Design review of the part shown in the three views and the two pictorial views. Dimensions are in mm from the part's minimum x, y and z. A direction names the side the tool comes from. Coordinates: 2 decimals unless noted, no trailing zeros. Loops run counter-clockwise (first coordinate to the right, second up) from the corner with the lowest first, then second, coordinate; pieces in that order, holes last. Notation, with made-up numbers: (-9, 38) -> (4, 38) arc R31 cw to (4, 67) -> close; hole circle Ø7 at (19.5, 14.25). An arc over 180 degrees is marked (long way). One line per item, written item: value. Start each with the question number.
1. Add section B-B on z = 14. Write out the cut boundary in (x, y).
2. Insertion check: pin 1 (1.5 mm diameter, centred on x = 21, z = 7, fed in from -Y); pin 2 (6 mm diameter, centred on x = 5, y = 28, fed in from +Z). Each pin has a flat end and moves straight along its axis. Give the tip position at first contact, or say it passes through.
3. Add section C-C on y = 21. Write out the cut boundary in (x, z).
4. Add section D-D on z = 31. Write out the cut boundary in (x, y).
5. For probe 1 along Y at (x, z) = (5.25, 14); probe 2 along X at (y, z) = (0.5, 32); probe 3 along Z at (x, y) = (16.75, 49.5), list the stretches that pass through material, from the lowest coordinate up.
6. Machinability: for the marked faces 1 and 2, which of the approach directions +Z, -Z, +X, -X, +Y, -Y give a long, thin tool a straight path to every point of the face, cutting with its end or side? Answer none if there is none.
7. Draft analysis for pull direction Y (two halves, no side actions). For the marked faces 3, 4 and 5, state which applies: pulls with the +Y half, pulls with the -Y half, needs draft (parallel to the pull), parting line crosses it, or undercut.
8. Add section A-A on x = 5.5. Write out the cut boundary in (y, z), plus the area to 3 significant figures.
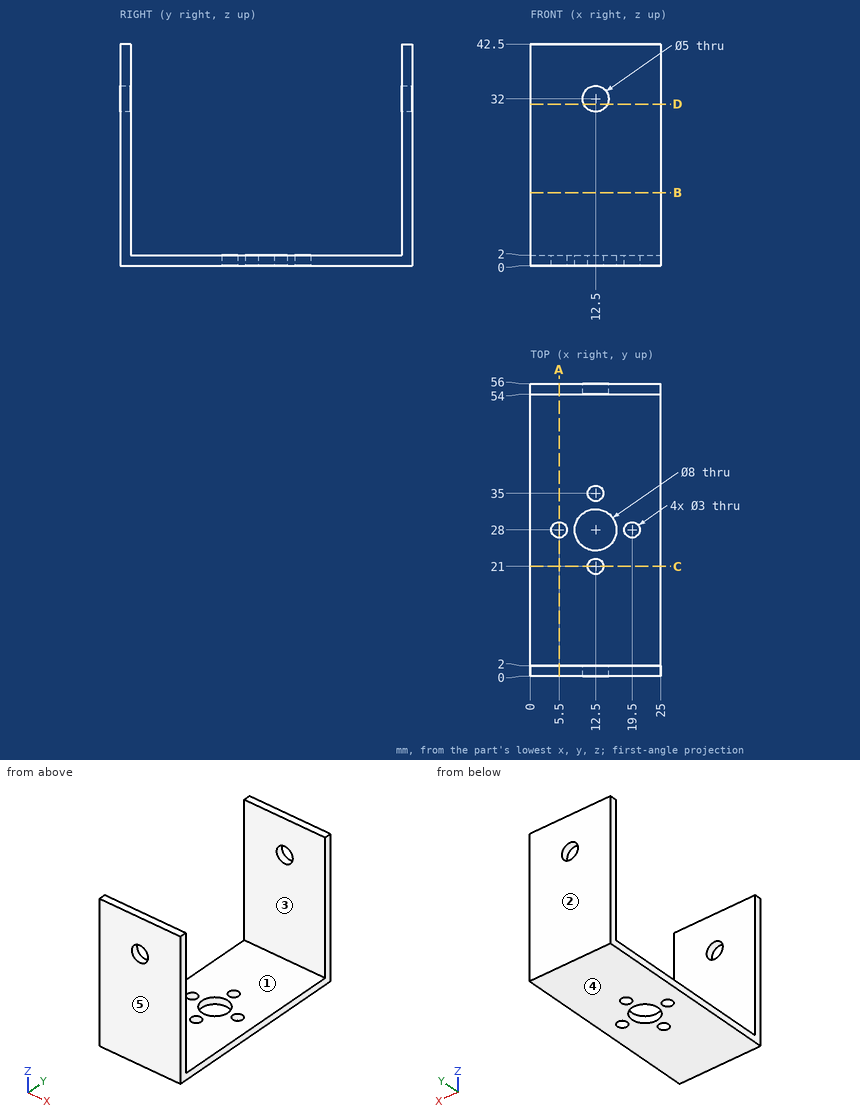
Worked answers:
1. outline: (0, 0) -> (25, 0) -> (25, 2) -> (0, 2) -> close; (0, 54) -> (25, 54) -> (25, 56) -> (0, 56) -> close
2. pin 1: stops at y = 0
2. pin 2: stops at z = 2
3. outline: (0, 0) -> (11, 0) -> (11, 2) -> (0, 2) -> close; (14, 0) -> (25, 0) -> (25, 2) -> (14, 2) -> close
4. outline: (0, 0) -> (10.21, 0) -> (10.21, 2) -> (0, 2) -> close; (0, 54) -> (10.21, 54) -> (10.21, 56) -> (0, 56) -> close; (14.79, 0) -> (25, 0) -> (25, 2) -> (14.79, 2) -> close; (14.79, 54) -> (25, 54) -> (25, 56) -> (14.79, 56) -> close
5. probe 1: y = 0 to 2, 54 to 56
5. probe 2: x = 0 to 10, 15 to 25
5. probe 3: z = 0 to 2
6. face 1: +Z, +X, -X
6. face 2: +Z, -Z, +X, -X, +Y
7. face 3: undercut
7. face 4: needs draft
7. face 5: pulls with the -Y half
8. outline: (0, 0) -> (26.5, 0) -> (26.5, 2) -> (2, 2) -> (2, 42.5) -> (0, 42.5) -> close; (29.5, 0) -> (56, 0) -> (56, 42.5) -> (54, 42.5) -> (54, 2) -> (29.5, 2) -> close
8. area: 268 mm²
